The drawing under review shows one solid part. Ordinate dimensions are in mm from its lowest x, y, z. A direction names the side the tool comes from. Round coordinates to 2 decimals unless told otherwise and drop trailing zeros. Order: outer loops, then holes, each group sorted by start corner. A loop starts at its lowest first (then second) coordinate and runs counter-clockwise, first axis right, second up. Notation, with made-up numbers: (11.25, -5.75) -> (65.25, -5.75) arc R23 cw to (65.25, 3.25) -> close; hole circle Ø6 at (57, 84). An arc over 180 degrees is marked (long way). Use a Markdown table: item, result. Add a question column.
1) Draft analysis for pull direction Y (two halves, no side actions). For the marked faces 1, 2 and 3, state which applies: pulls with the +Y half, pulls with the -Y half, needs draft (parallel to the pull), parting line crosses it, or undercut.
2) Consider section D-D (z = 34). State the section outline as (x, y) points.
3) Consider section A-A (x = 178). State the section outline as (y, z) points, plus the area to 3 significant figures.
4) Clearance check with flat-ended pins moving along their axes: P1, Ø10, axis at y = 49.5, z = 29.5, coming from the -X side; P2, Ø8, axis at x = 157.5, z = 47.55, coming from the -Y side. State where each tip first meets the part, or that it passes through.
5) Consider section C-C (x = 157.5). State the section outline as (y, z) points, plus the area to 3 significant figures.
6) Machinability: for the marked faces 4 and 5, which of the approach directions +Z, -Z, +X, -X, +Y, -Y give a long, thin tool a straight path to every point of the face, cutting with its end or side? Answer none if there is none.
7) Consider section B-B (y = 70.5). State the section outline as (x, z) points.
8) Wall thickness on line 1 along Z through (x, y) = (157.5, 81.5); line 2 along Z through (x, y) = (10, 1); line 3 along X through (y, z) = (40.5, 39): over which ranges is each line inside the solid? List them lowest first. Write a range as [from, to].
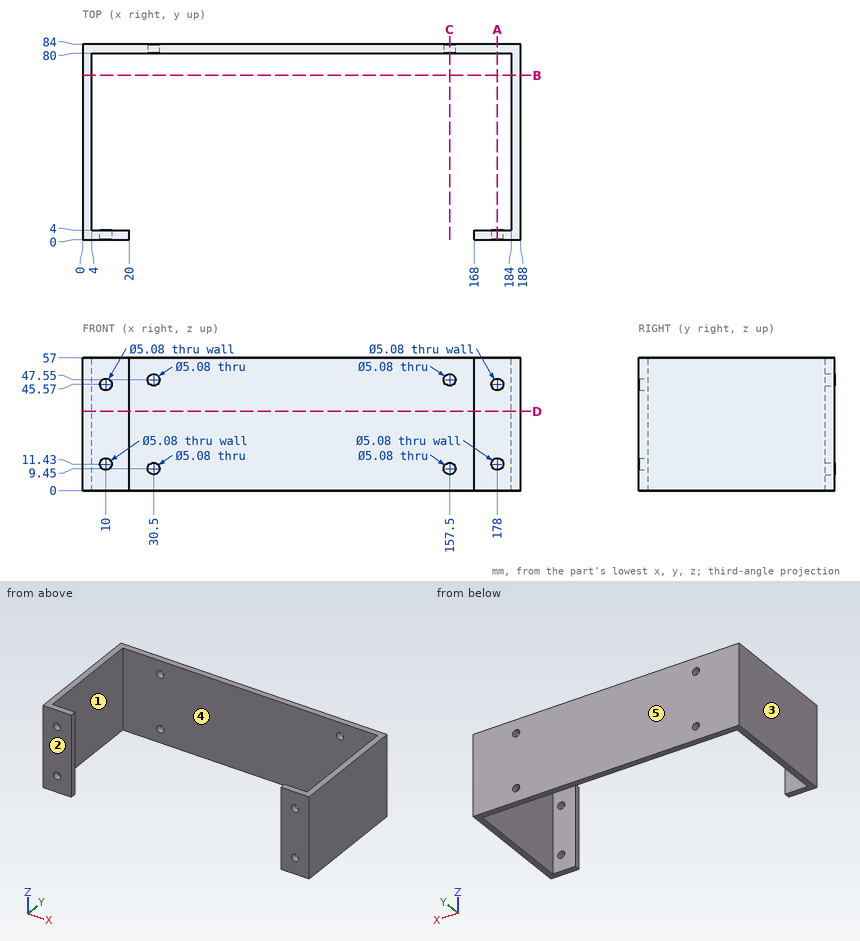
Results list:
| question | item | result |
|---|---|---|
| 1 | face 1 | undercut |
| 1 | face 2 | pulls with the -Y half |
| 1 | face 3 | needs draft |
| 2 | outline | (0, 0) -> (20, 0) -> (20, 4) -> (4, 4) -> (4, 80) -> (184, 80) -> (184, 4) -> (168, 4) -> (168, 0) -> (188, 0) -> (188, 84) -> (0, 84) -> close |
| 3 | outline | (0, 0) -> (4, 0) -> (4, 8.89) -> (0, 8.89) -> close; (0, 13.97) -> (4, 13.97) -> (4, 43.03) -> (0, 43.03) -> close; (0, 48.11) -> (4, 48.11) -> (4, 57) -> (0, 57) -> close; (80, 0) -> (84, 0) -> (84, 57) -> (80, 57) -> close |
| 3 | area | 415 mm2 |
| 4 | P1 | x = 0 |
| 4 | P2 | y = 80 |
| 5 | outline | (80, 0) -> (84, 0) -> (84, 6.91) -> (80, 6.91) -> close; (80, 11.99) -> (84, 11.99) -> (84, 45.01) -> (80, 45.01) -> close; (80, 50.09) -> (84, 50.09) -> (84, 57) -> (80, 57) -> close |
| 5 | area | 187 mm2 |
| 6 | face 4 | +Z, -Z |
| 6 | face 5 | +Z, -Z, +X, -X, +Y |
| 7 | outline | (0, 0) -> (4, 0) -> (4, 57) -> (0, 57) -> close; (184, 0) -> (188, 0) -> (188, 57) -> (184, 57) -> close |
| 8 | line 1 | [0, 6.91], [11.99, 45.01], [50.09, 57] |
| 8 | line 2 | [0, 8.89], [13.97, 43.03], [48.11, 57] |
| 8 | line 3 | [0, 4], [184, 188] |
